from build123d import *

# Parameters (mm, degrees)
SKIZZE1_W                       = 90
SKIZZE1_H                       = 50
AUFSATZ_LINEAR_AUSTRAGEN1_DEPTH = 7.5
SKIZZE2_R                       = 1
SCHNITT_LINEAR_AUSTRAGEN1_DEPTH = 53.021630117
SCHNITT_LINEAR_AUSTRAGEN2_DEPTH = 2.7
SKIZZE6_W                       = 13
SKIZZE6_H                       = 4
SCHNITT_LINEAR_AUSTRAGEN5_DEPTH = 94.70832407
M3_GEWINDEBOHRUNG1_D            = 2.5


with BuildPart() as part:
    # Skizze1 → Aufsatz-Linear austragen1 (new body)
    with BuildSketch(Plane(origin=(0, 0, 0), x_dir=(1, 0, 0), z_dir=(0, 1, 0))):
        Rectangle(SKIZZE1_W, SKIZZE1_H)
    extrude(amount=AUFSATZ_LINEAR_AUSTRAGEN1_DEPTH)

    # Skizze2 → Schnitt-Linear austragen1 (cut, through all)
    with BuildSketch(Plane(origin=(0, 7.5, 0), x_dir=(1, 0, 0), z_dir=(0, 1, 0))):
        with Locations(Location((-35, 14.5, 0), (0, 0, 270))):
            Circle(SKIZZE2_R)
        with Locations(Location((-15, 14.5, 0), (0, 0, 270))):
            Circle(SKIZZE2_R)
        with Locations(Location((-35, -14.5, 0), (0, 0, 90))):
            Circle(SKIZZE2_R)
        with Locations(Location((-15, -14.5, 0), (0, 0, 90))):
            Circle(SKIZZE2_R)
        with BuildLine():
            Line((-10, 9.5), (40, 9.5))
            ThreePointArc((40, 9.5), (41.5, 8), (40, 6.5))
            Line((40, 6.5), (-10, 6.5))
            ThreePointArc((-10, 6.5), (-11.5, 8), (-10, 9.5))
        make_face()
        with BuildLine():
            Line((-10, -9.5), (40, -9.5))
            ThreePointArc((40, -9.5), (41.5, -8), (40, -6.5))
            Line((40, -6.5), (-10, -6.5))
            ThreePointArc((-10, -6.5), (-11.5, -8), (-10, -9.5))
        make_face()
    extrude(amount=-SCHNITT_LINEAR_AUSTRAGEN1_DEPTH, mode=Mode.SUBTRACT)

    # Skizze3 → Schnitt-Linear austragen2 (cut)
    with BuildSketch(Plane(origin=(0, 7.5, 0), x_dir=(1, 0, 0), z_dir=(0, 1, 0))):
        with BuildLine():
            Line((-10, 11.2), (40, 11.2))
            ThreePointArc((40, 11.2), (43.2, 8), (40, 4.8))
            Line((40, 4.8), (-10, 4.8))
            ThreePointArc((-10, 4.8), (-13.2, 8), (-10, 11.2))
        make_face()
        with BuildLine():
            Line((-10, -11.2), (40, -11.2))
            ThreePointArc((40, -11.2), (43.2, -8), (40, -4.8))
            Line((40, -4.8), (-10, -4.8))
            ThreePointArc((-10, -4.8), (-13.2, -8), (-10, -11.2))
        make_face()
    extrude(amount=-SCHNITT_LINEAR_AUSTRAGEN2_DEPTH, mode=Mode.SUBTRACT)

    # Skizze6 → Schnitt-Linear austragen5 (cut, through all)
    with BuildSketch(Plane.ZY.offset(45)):
        with Locations((-23.5, 2)):
            Rectangle(SKIZZE6_W, SKIZZE6_H)
        with Locations((23.5, 2)):
            Rectangle(SKIZZE6_W, SKIZZE6_H)
    extrude(amount=-SCHNITT_LINEAR_AUSTRAGEN5_DEPTH, mode=Mode.SUBTRACT)

    # M3 Gewindebohrung1 (through all)
    with Locations(Plane(origin=(0, 7.5, 0), x_dir=(1, 0, 0), z_dir=(0, 1, 0))):
        with Locations((-25, 14.5), (-25, -14.5)):
            Hole(M3_GEWINDEBOHRUNG1_D / 2)


solid = part.part
Can you work these out from the model? Positions are in its coordinate system, mm. A direction names the side the tool comes from. Coordinates: 2 decimals unless noted, no trailing zeros. Write each loop counter-clockwise with the first axis right and the second up, starting at its lowest first coordinate (ties: lowest second). Pieces come first, ordered by that corner, then holes.
Q1. For P1, Ø4, axis at x = 11, y = 1.5, coming from the -Z side; P2, Ø1.2, axis at x = -16.5, y = 2.5, coming from the +Z side; P3, Ø3, axis at x = 24.5, z = -9.5, coming from the +Y side, each with a flat end and sliding along its axis, tell me the tip position at first contact or that it passes through.
Results found:
P1: stops at z = -17
P2: stops at z = 17
P3: stops at y = 4.8
Q2. If we mould it in two halves opening along X, with no side actions, what happens to faces 6 (the face through (45, 4, 0)), 7 (the face through (-15.89, 3.8, -14.04)), 8 (the face through (-1, 2, -17))? For each: +X half, -X half, draft (parallel to the pull), parting line (faces both ways), or undercut.
Results found:
face 6: +X half
face 7: undercut
face 8: draft
Q3. Imagine slicing it at C-C, the plane y = 3. Count the separate pieces of the cut face and the enclosed holes in it, plus the area to 3 significant figures.
Results found:
separate pieces: 1
enclosed holes: 8
area: 2,720 mm2
Q4. Please list where these lines run through material, in increasing order: L1, parallel to Z at x = 31, y = 6.25; L2, parallel to Z at x = 18.5, y = 4.75; L3, parallel to X at y = 5.25, z = 14.5.
Results found:
L1: z = -25 to -11.2, -4.8 to 4.8, 11.2 to 25
L2: z = -25 to -9.5, -6.5 to 6.5, 9.5 to 25
L3: x = -45 to -36, -34 to -26.25, -23.75 to -16, -14 to 45
Q5. Imagine slicing it at B-B, the plane z = -8. List the corners of the cut face in (x, y) for me, plus the area to 3 significant figures.
Results found:
outline: (-45, 0) - (-11.5, 0) - (-11.5, 4.8) - (-13.2, 4.8) - (-13.2, 7.5) - (-45, 7.5) - close; (41.5, 0) - (45, 0) - (45, 7.5) - (43.2, 7.5) - (43.2, 4.8) - (41.5, 4.8) - close
area: 268 mm2
Q6. Imagine slicing it at A-A, the plane x = 0.5. List the corners of the cut face in (y, z) for me.
Results found:
outline: (0, -17) - (4, -17) - (4, -25) - (7.5, -25) - (7.5, -11.2) - (4.8, -11.2) - (4.8, -9.5) - (0, -9.5) - close; (0, -6.5) - (4.8, -6.5) - (4.8, -4.8) - (7.5, -4.8) - (7.5, 4.8) - (4.8, 4.8) - (4.8, 6.5) - (0, 6.5) - close; (0, 9.5) - (4.8, 9.5) - (4.8, 11.2) - (7.5, 11.2) - (7.5, 25) - (4, 25) - (4, 17) - (0, 17) - close
Q7. Which directions (+Z, -Z, +X, -X, +Y, -Y) give clear straight access to the entire face, cutting with the end or side of a thin tool? Please do faces 1 (the face through (15, 4.8, -10)), 2 (the face through (-1, 6, -25)), 3 (the face through (-1, 7.5, 0)), 4 (the face through (-1, 4, 21)), 5 (the face through (15, 2, 9.5)).
Results found:
face 1: +Y
face 2: -Z, +X, -X, +Y, -Y
face 3: +Z, -Z, +X, -X, +Y
face 4: +Z, +X, -X, -Y
face 5: +Y, -Y
Q8. Imagine slicing it at D-D, the plane z = 14.5. List the corners of the cut face in (x, y) for me.
Results found:
outline: (-45, 0) - (-36, 0) - (-36, 7.5) - (-45, 7.5) - close; (-34, 0) - (-26.25, 0) - (-26.25, 7.5) - (-34, 7.5) - close; (-23.75, 0) - (-16, 0) - (-16, 7.5) - (-23.75, 7.5) - close; (-14, 0) - (45, 0) - (45, 7.5) - (-14, 7.5) - close
